from build123d import *

# Parameters (mm, degrees)
SKETCH1_R           = 15.75
BOSS_EXTRUDE1_DEPTH = 109
CHAMFER1_SIZE       = 2
CHAMFER1_SIZE2      = 10.791034349
SKETCH2_R           = 4.958965651
BOSS_EXTRUDE2_DEPTH = 10
BOSS_EXTRUDE3_DEPTH = 2.3
BOSS_EXTRUDE4_DEPTH = 111
SKETCH5_R           = 16.5
BOSS_EXTRUDE5_DEPTH = 2


with BuildPart() as part:
    # Sketch1 → Boss-Extrude1 (new body)
    with BuildSketch(Plane(origin=(0, 0, 0), x_dir=(1, 0, 0), z_dir=(0, 1, 0))):
        with Locations(Location((0, 0, 0), (0, 0, 270))):
            Circle(SKETCH1_R)
    extrude(amount=BOSS_EXTRUDE1_DEPTH)

    # Chamfer1
    chamfer1_edges = [part.edges().sort_by_distance(p)[0] for p in [
        (0, 109, -15.75),
    ]]
    chamfer1_side = [part.faces().sort_by_distance(p)[0] for p in [
        (0, 54.5, -15.75),
    ]]
    chamfer(chamfer1_edges, length=CHAMFER1_SIZE, length2=CHAMFER1_SIZE2, reference=chamfer1_side[0])

    # Sketch2 → Boss-Extrude2 (add)
    with BuildSketch(Plane(origin=(0, 109, 0), x_dir=(1, 0, 0), z_dir=(0, 1, 0))):
        with Locations(Location((0, 0, 0), (0, 0, 90))):
            Circle(SKETCH2_R)
    extrude(amount=BOSS_EXTRUDE2_DEPTH)

    # Sketch3 → Boss-Extrude3 (add)
    with BuildSketch(Plane.XZ):
        with BuildLine():
            Line((-17, 12), (-17, -12))
            ThreePointArc((-17, -12), (-16.155417528, -15.577708764), (-13.8, -18.4))
            ThreePointArc((-13.8, -18.4), (0, -23), (13.8, -18.4))
            ThreePointArc((13.8, -18.4), (16.155417528, -15.577708764), (17, -12))
            Line((17, -12), (17, 12))
            ThreePointArc((17, 12), (16.155417528, 15.577708764), (13.8, 18.4))
            ThreePointArc((13.8, 18.4), (0, 23), (-13.8, 18.4))
            ThreePointArc((-13.8, 18.4), (-16.155417528, 15.577708764), (-17, 12))
        make_face()
    extrude(amount=BOSS_EXTRUDE3_DEPTH)

    # Sketch4 → Boss-Extrude4 (add)
    with BuildSketch(Plane.XZ.offset(2.3)):
        Polygon((0.75, 0.75), (7.5, 0.75), (7.5, -0.75), (0.75, -0.75), (0.75, -7.5), (-0.75, -7.5), (-0.75, -0.75), (-7.5, -0.75), (-7.5, 0.75), (-0.75, 0.75), (-0.75, 7.5), (0.75, 7.5), align=None)
    extrude(amount=BOSS_EXTRUDE4_DEPTH)

    # Sketch5 → Boss-Extrude5 (add)
    with BuildSketch(Plane.XZ.offset(113.3)):
        with Locations(Location((0, 0, 0), (0, 0, 270))):
            Circle(SKETCH5_R)
    extrude(amount=BOSS_EXTRUDE5_DEPTH)


solid = part.part
The model under review builds one solid part; all positions refer to its coordinate system, in mm. A direction names the side the tool comes from. Round coordinates to 2 decimals unless told otherwise and drop trailing zeros. Loops run counter-clockwise (first coordinate to the right, second up) from the corner with the lowest first, then second, coordinate; pieces in that order, holes last. Notation, with made-up numbers: M -27,6.5 L 11,6.5 A28 cw 11,29.5 Z; hole C -7,38.25 d11. An arc over 180 degrees is marked long. Answer as a JSON object with one key per item and string values.
Item 1: We need section B-B, the plane y = 34.5. State the section outline as (x, z) points.
Check sheet entries:
{"outline": "C 0,0 d31.5"}
Item 2: For line 1 along Y through (x, z) = (-8.5, -14); line 2 along Y through (x, z) = (-2.5, 2); line 3 along X through (y, z) = (31.5, 1), list the stretches that pass through material, from the lowest coordinate up.
Check sheet entries:
{"line 1": "-115.3 to -113.3, -2.3 to 0", "line 2": "-115.3 to -113.3, -2.3 to 119", "line 3": "-15.72 to 15.72"}
Item 3: The part is to be moulded in two halves that separate along Y. For faces 1 (the face through (-5.353, 108.903, -1.189)), 2 (the face through (-3, -113.3, -3)), 3 (the face through (0, -1, -23)), say which applies: +Y half, -Y half, draft (parallel to the pull), parting line (faces both ways), or undercut.
Check sheet entries:
{"face 1": "+Y half", "face 2": "undercut", "face 3": "draft"}
Item 4: Tool access review of faces 4 (the face through (0.75, -57, -4)), 5 (the face through (15.616, 52.751, -2.05)), 6 (the face through (-4, -57, -0.75)): name each direction out of +Z, -Z, +X, -X, +Y, -Y from which nothing blocks a thin tool from reaching the whole face with its end or side.
Check sheet entries:
{"face 4": "-Z, +X", "face 5": "+Y", "face 6": "-Z, -X"}
Item 5: We need section A-A, the plane y = -26. State the section outline as (x, z) points.
Check sheet entries:
{"outline": "M -7.5,-0.75 L -0.75,-0.75 L -0.75,-7.5 L 0.75,-7.5 L 0.75,-0.75 L 7.5,-0.75 L 7.5,0.75 L 0.75,0.75 L 0.75,7.5 L -0.75,7.5 L -0.75,0.75 L -7.5,0.75 Z"}
Item 6: Clearance check with flat-ended pins moving along their axes: P1, Ø2, axis at y = -83.5, z = 5, coming from the +X side; P2, Ø2, axis at x = -2.5, y = -43, coming from the -Z side; P3, Ø3.5, axis at y = -31.5, z = 3.5, coming from the -X side. State where each tip first meets the part, or that it passes through.
Check sheet entries:
{"P1": "x = 0.75", "P2": "z = -0.75", "P3": "x = -0.75"}
